The listing builds one solid part. Answer for the finished solid, in the listing's coordinates (mm). A direction names the side the tool comes from. Round coordinates to 2 decimals unless told otherwise and drop trailing zeros. Write each loop counter-clockwise with the first axis right and the second up, starting at its lowest first coordinate (ties: lowest second). Pieces come first, ordered by that corner, then holes.
from build123d import *

# Parameters (mm, degrees)
ESQUISSE1_W             = 20
ESQUISSE1_H             = 85
BOSS_EXTRU_1_DEPTH      = 15
ESQUISSE2_R             = 2.5
ENL_V_MAT_EXTRU_1_DEPTH = 15


with BuildPart() as part:
    # Esquisse1 → Boss.-Extru.1 (new body)
    with BuildSketch(Plane.XY):
        with Locations((10, 42.5)):
            Rectangle(ESQUISSE1_W, ESQUISSE1_H)
    extrude(amount=BOSS_EXTRU_1_DEPTH)

    # Esquisse2 → Enlèv. mat.-Extru.1 (cut)
    with BuildSketch(Plane.XY.offset(15)):
        with Locations((10, 79)):
            Circle(ESQUISSE2_R)
        with BuildLine():
            Line((6.75, 8), (6.75, 69))
            ThreePointArc((6.75, 69), (10, 72.25), (13.25, 69))
            Line((13.25, 69), (13.25, 8))
            ThreePointArc((13.25, 8), (10, 4.75), (6.75, 8))
        make_face()
    extrude(amount=-ENL_V_MAT_EXTRU_1_DEPTH, mode=Mode.SUBTRACT)


solid = part.part
1. Section A-A on x = 10 is taken. Determine the outline of the cut face in (y, z).
Geometry says:
outline: (0, 0) - (4.75, 0) - (4.75, 15) - (0, 15) - close; (72.25, 0) - (76.5, 0) - (76.5, 15) - (72.25, 15) - close; (81.5, 0) - (85, 0) - (85, 15) - (81.5, 15) - close
2. Section D-D on y = 24.5 is taken. Determine the outline of the cut face in (x, z).
Geometry says:
outline: (0, 0) - (6.75, 0) - (6.75, 15) - (0, 15) - close; (13.25, 0) - (20, 0) - (20, 15) - (13.25, 15) - close
3. A tool of negligible diameter and unlimited length cuts with its end or side. For faces 1 (the face through (9.93, 72.25, 7.6)), 2 (the face through (20, 42, 7)), from which of +Z, -Z, +X, -X, +Y, -Y can it reach the whole face along a straight path? Write none if from no direction.
Geometry says:
face 1: +Z, -Z
face 2: +Z, -Z, +X, +Y, -Y
4. Straight lines are drawn through the part: line 1 along Y through (x, z) = (10, 4.5); line 2 along X through (y, z) = (23, 12.5); line 3 along Y through (x, z) = (9.5, 4). For each, find the intervals that lie inside material, in ascending order.
Geometry says:
line 1: y = 0 to 4.75, 72.25 to 76.5, 81.5 to 85
line 2: x = 0 to 6.75, 13.25 to 20
line 3: y = 0 to 4.79, 72.21 to 76.55, 81.45 to 85
5. For a pull along Y with two mould halves and no side action, classify faces 3 (the face through (10, 85, 7)), 4 (the face through (11.15, 76.78, 7.6)), 5 (the face through (5, 43, 15)) as released by +Y, released by -Y, zero draft, split by the parting line, or undercut.
Geometry says:
face 3: released by +Y
face 4: undercut
face 5: zero draft
6. Section B-B on y = 79 is taken. Determine the outline of the cut face in (x, z), plus the area to 3 significant figures.
Geometry says:
outline: (0, 0) - (7.5, 0) - (7.5, 15) - (0, 15) - close; (12.5, 0) - (20, 0) - (20, 15) - (12.5, 15) - close
area: 225 mm2
7. Section C-C on z = 8 is taken. Determine the outline of the cut face in (x, y).
Geometry says:
outline: (0, 0) - (20, 0) - (20, 85) - (0, 85) - close; hole (6.75, 8) arc R3.25 ccw to (13.25, 8) - (13.25, 69) arc R3.25 ccw to (6.75, 69) - close; hole circle Ø5 at (10, 79)
